from build123d import *

# Parameters (mm, degrees)
F0_W     = 101.6
F0_H     = 50.8
F0_R     = 1.1303
F0_W_2   = 41.275
F0_H_2   = 20.828
F1_DEPTH = 6.35
F3_DEPTH = 50.801
F4_W     = 6.35
F4_H     = 50.8
F5_DEPTH = 59.69
F7_DEPTH = 6.35
F9_DEPTH = 6.35


with BuildPart() as f1:
    # F0 (on Top) → F1 (new body)
    with BuildSketch(Plane.XY):
        with Locations((50.8, 25.4)):
            Rectangle(F0_W, F0_H)
        with Locations((41.5798, 20.574)):
            Circle(F0_R, mode=Mode.SUBTRACT)
        with Locations((66.3575, 25.4)):
            Rectangle(F0_W_2, F0_H_2, mode=Mode.SUBTRACT)
        with Locations((91.1098, 20.574)):
            Circle(F0_R, mode=Mode.SUBTRACT)
        with Locations((41.5798, 30.226)):
            Circle(F0_R, mode=Mode.SUBTRACT)
        with Locations((91.1098, 30.226)):
            Circle(F0_R, mode=Mode.SUBTRACT)
    extrude(amount=F1_DEPTH)

    # F2 (on face) → F3 (cut, through all)
    with BuildSketch(Plane.XZ):
        Polygon((0, 3.333318), (0, 0), (38.1, 0), align=None)
    extrude(amount=-F3_DEPTH, mode=Mode.SUBTRACT)

    # F4 (on face) → F5 (join)
    with BuildSketch(Plane(origin=(0, 0, 0), x_dir=(1, 0, 0), z_dir=(0, 0, -1))):
        with Locations((98.425, -25.4)):
            Rectangle(F4_W, F4_H)
    extrude(amount=F5_DEPTH)

    # F6 (on face) → F7 (cut, through all)
    with BuildSketch(Plane(origin=(95.25, 0, 0), x_dir=(0, -1, 0), z_dir=(-1, 0, 0))):
        with BuildLine():
            Line((-28.575, -29.21), (-28.575, -59.69))
            Line((-28.575, -59.69), (-22.225, -59.69))
            Line((-22.225, -59.69), (-22.225, -29.21))
            ThreePointArc((-22.225, -29.21), (-25.4, -26.035), (-28.575, -29.21))
        make_face()
    extrude(amount=-F7_DEPTH, mode=Mode.SUBTRACT)

    # F8 (on face) → F9 (cut, through all)
    with BuildSketch(Plane.YZ.offset(101.6)):
        Polygon((50.8, -59.69), (50.8, -2.54), (33.02, -59.69), align=None)
        Polygon((0, -2.54), (0, -59.69), (17.78, -59.69), align=None)
    extrude(amount=-F9_DEPTH, mode=Mode.SUBTRACT)


solid = f1.part
Input: part model. Units: mm. Frame: model coordinates. A direction names the side the tool comes from. Coordinates: 2 decimals unless noted, no trailing zeros. Order: outer loops, then holes, each group sorted by start corner. A loop starts at its lowest first (then second) coordinate and runs counter-clockwise, first axis right, second up. Notation, with made-up numbers: M 48.25,28.5 L 80.25,28.5 A22 ccw 80.25,40.5 Z; hole C -21.5,3.5 d2. An arc over 180 degrees is marked long. One line per question, with ' | ' between items.
Item 1: Section A-A (y = 25.4). Output: boundary loops of the cut face in (x, z) (3 decimals).
Geometry results:
outline: M 0,3.333 L 38.1,0 L 45.72,0 L 45.72,6.35 L 0,6.35 Z; M 86.995,0 L 95.25,0 L 95.25,-26.035 L 101.6,-26.035 L 101.6,6.35 L 86.995,6.35 Z
Item 2: Reachability of faces 1 (the flat face through (45.72, 25, 3)), 2 (the flat face through (95.25, 26, -23)), 3 (the flat face through (98, 22.225, -45)) from +Z, -Z, +X, -X, +Y, -Y: full face, straight path, thin tool, end or side. Return the list, or none.
Geometry results:
face 1: +Z, -Z | face 2: -Z, -X, +Y, -Y | face 3: -Z, +X, -X
Item 3: Pin query (flat end, axial travel): pin 1 (5 mm diameter, centred on x = 98.5, z = -50.5, fed in from +Y); pin 2 (5 mm diameter, centred on y = 20, z = -36.5, fed in from -X); pin 3 (5 mm diameter, centred on x = 97.5, z = -42.5, fed in from -Y). Return the tip coordinate at first contact, or that it passes through.
Geometry results:
pin 1: stops at y = 36.66 | pin 2: stops at x = 95.25 | pin 3: stops at y = 11.65
Item 4: Section C-C (z = -51). Output: boundary loops of the cut face in (x, y) (3 decimals).
Geometry results:
outline: M 95.25,15.076 L 101.6,15.076 L 101.6,22.225 L 95.25,22.225 Z; M 95.25,28.575 L 101.6,28.575 L 101.6,35.724 L 95.25,35.724 Z
Item 5: Ray query, line 1 along X through (y, z) = (13, -37.5); line 2 along Z through (x, y) = (94, 25); line 3 along Z through (x, y) = (12, 18.5). Return the intervals inside material, ascending.
Geometry results:
line 1: x = 95.25 to 101.6 | line 2: z = 0 to 6.35 | line 3: z = 2.28 to 6.35
Item 6: Draft query along X for faces 4 (the flat face through (66, 14.986, 3)), 5 (the flat face through (98, 20, -59.69)), 6 (the cylindrical face through (42.101, 29.223, 3.131)), 7 (the flat face through (0, 25, 5)). Return one class per face: released by +X, released by -X, zero draft, split by the parting line, or undercut.
Geometry results:
face 4: undercut | face 5: zero draft | face 6: undercut | face 7: released by -X
Item 7: Section B-B (x = 84.5). Output: boundary loops of the cut face in (y, z), then the cut area to 3 significant figures.
Geometry results:
outline: M 0,0 L 14.99,0 L 14.99,6.35 L 0,6.35 Z; M 35.81,0 L 50.8,0 L 50.8,6.35 L 35.81,6.35 Z | area: 190 mm^2
Item 8: Section D-D (y = 11). Output: boundary loops of the cut face in (x, z), then the cut area to 3 significant figures.
Geometry results:
outline: M 0,3.33 L 38.1,0 L 95.25,0 L 95.25,-37.9 L 101.6,-37.9 L 101.6,6.35 L 0,6.35 Z | area: 822 mm^2
